For this review, take the finished solid that the model builds, in its own axes (mm). Face numbers are marked on the shaded views. Round coordinates to 2 decimals unless told otherwise and drop trailing zeros. Order: outer loops, then holes, each group sorted by start corner. A loop starts at its lowest first (then second) coordinate and runs counter-clockwise, first axis right, second up. Notation, with made-up numbers: M -20.75,-37 L 7.25,-37 A11 ccw 7.25,-30 Z; hole C 58.5,4 d4. An arc over 180 degrees is marked long. Use a Markdown table: item, result.
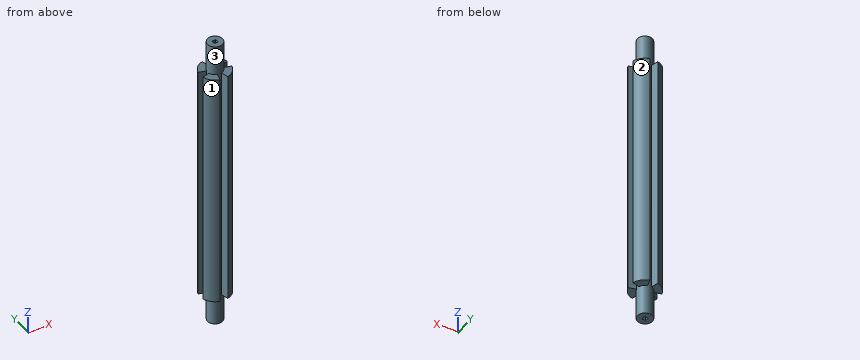
Autodesk Inventor part; units mm, degrees
ref_plane "YZ Plane" through (0, 0, 0) normal (1, 0, 0) x (0, 1, 0)
ref_plane "XZ Plane" through (0, 0, 0) normal (0, 1, 0) x (-1, 0, 0)
ref_plane "XY Plane" through (0, 0, 0) normal (0, 0, 1) x (1, 0, 0)
sketch "Sketch1" plane through (0, 0, 0) normal (0, 0, 1) x (1, 0, 0)
  circle A0 centre (0, 0) radius 6.35
  line L0 (-1.5875, -1.5875) -> (1.5875, -1.5875)
  line L1 (1.5875, -1.5875) -> (1.5875, 1.5875)
  line L2 (1.5875, 1.5875) -> (-1.5875, 1.5875)
  line L3 (-1.5875, 1.5875) -> (-1.5875, -1.5875)
  line L4 (-1.5875, -1.5875) -> (1.5875, 1.5875) construction
  line L5 (1.5875, -1.5875) -> (-1.5875, 1.5875) construction
  dimension "d0" = 12.7
  dimension "d3" = 3.175
  dimension "d4" = 3.175
extrude "Extrusion1" add sketch "Sketch1" along normal blind 254 contours A0 | L3 L2 L1 L0
extrude "Extrusion2" cut sketch "Sketch1" along normal blind 254 contours L3 L2 L1 L0
ref_plane "Work Plane1" through (0, 0, 25.4) normal (0, 0, -1) x (-1, 0, 0)
sketch "Sketch2" plane through (0, 0, 25.4) normal (0, 0, -1) x (-1, 0, 0)
  circle A0 centre (0, 0) radius 10.16
  line L0 (0, 0) -> (-12.2827, 3.2288)
  circle A1 centre (0, 0) radius 6.35
  line L1 (-12.2827, -3.2288) -> (0, 0)
  arc A2 (-3.2288, 12.2827) -> (-12.2827, 3.2288) centre (0, 0) ccw
  arc A3 (12.2827, 3.2288) -> (3.2288, 12.2827) centre (0, 0) ccw
  arc A4 (-12.2827, -3.2288) -> (-3.2288, -12.2827) centre (0, 0) ccw
  arc A5 (3.2288, -12.2827) -> (12.2827, -3.2288) centre (0, 0) ccw
  line L2 (0, 0) -> (-3.2288, -12.2827)
  line L3 (3.2288, -12.2827) -> (0, 0)
  line L4 (0, 0) -> (12.2827, -3.2288)
  line L5 (12.2827, 3.2288) -> (0, 0)
  line L6 (0, 0) -> (3.2288, 12.2827)
  line L7 (-3.2288, 12.2827) -> (0, 0)
  point P0 (-1.6144, -6.1414)
  point P1 (-6.1414, -1.6144)
  point P2 (6.1414, -1.6144)
  point P3 (1.6144, -6.1414)
  point P4 (1.6144, 6.1414)
  point P5 (6.1414, 1.6144)
  point P6 (-6.1414, 1.6144)
  point P7 (-1.6144, 6.1414)
  dimension "d11" = 20.32
  dimension "d20" = 360
extrude "Extrusion4" add sketch "Sketch2" against normal blind 203.2 contours L5 A1 L6 A0 | A0 L6 A3 L5 | L4 A5 L3 A0 | A0 L3 A1 L4 | L7 A1 L0 A0 | A0 L0 A2 L7 | L2 A4 L1 A0 | A0 L1 A1 L2
properties part number "Nicoles_Roomba_Blade_Axle"
Q1. Wall thickness on line 1 along X through (y, z) = (-1.5, 44); line 2 along Z through (x, y) = (-2.5, -7.5); line 3 along X through (y, z) = (8.75, 89.5): over which ranges is each line inside the solid? List them lowest first. Write a range as [from, to].
Determined:
| item | result |
|---|---|
| line 1 | x = [-6.17, -1.59], [1.59, 6.17] |
| line 2 | z = [25.4, 228.6] |
| line 3 | x = [-9.2, -2.3], [2.3, 9.2] |
Q2. Clearance check with flat-ended pins moving along their axes: pin 1 (11.5 mm diameter, centred on x = 6, y = -5, fed in from +Z); pin 2 (1.5 mm diameter, centred on y = 9, z = 78.5, fed in from -X); pin 3 (1 mm diameter, centred on y = 0.5, z = 160, fed in from -X); pin 4 (1 mm diameter, centred on x = 0.5, z = 69, fed in from +Y). State where each tip first meets the part, or that it passes through.
Determined:
| item | result |
|---|---|
| pin 1 | stops at z = 254 |
| pin 2 | stops at x = -9.66 |
| pin 3 | stops at x = -6.35 |
| pin 4 | stops at y = 6.35 |
Q3. Draft analysis for pull direction Y (two halves, no side actions). For the marked faces 1, 2 and 3, state which applies: pulls with the +Y half, pulls with the -Y half, needs draft (parallel to the pull), parting line crosses it, or undercut.
Determined:
| item | result |
|---|---|
| face 1 | pulls with the -Y half |
| face 2 | pulls with the +Y half |
| face 3 | undercut |
Q4. Add section A-A (z = 93). Write out the cut boundary in (x, y).
Determined:
| item | result |
|---|---|
| outline | M -12.28,-3.23 A12.7 ccw -3.23,-12.28 L -1.61,-6.14 A6.35 ccw 1.61,-6.14 L 3.23,-12.28 A12.7 ccw 12.28,-3.23 L 6.14,-1.61 A6.35 ccw 6.14,1.61 L 12.28,3.23 A12.7 ccw 3.23,12.28 L 1.61,6.14 A6.35 ccw -1.61,6.14 L -3.23,12.28 A12.7 ccw -12.28,3.23 L -6.14,1.61 A6.35 ccw -6.14,-1.61 Z; hole M -1.59,-1.59 L 1.59,-1.59 L 1.59,1.59 L -1.59,1.59 Z |
Q5. Add section B-B (y = 8.5). Write out the cut boundary in (x, z).
Determined:
| item | result |
|---|---|
| outline | M -9.44,25.4 L -2.23,25.4 L -2.23,228.6 L -9.44,228.6 Z; M 2.23,25.4 L 9.44,25.4 L 9.44,228.6 L 2.23,228.6 Z |
Q6. Add section C-C (y = -9.5). Write out the cut boundary in (x, z).
Determined:
| item | result |
|---|---|
| outline | M -8.43,25.4 L -2.5,25.4 L -2.5,228.6 L -8.43,228.6 Z; M 2.5,25.4 L 8.43,25.4 L 8.43,228.6 L 2.5,228.6 Z |
